```python
from build123d import *

# Parameters (mm, degrees)
SKETCH_1_R          = 1.5
EXTRUDE_1_DEPTH     = 3
CUT_EXTRUDE_1_DEPTH = 182.132548152
FILLET_1_R          = 2


with BuildPart() as part:
    # 草图1 → 凸台-拉伸1 (new body)
    with BuildSketch(Plane(origin=(0, 0, 0), x_dir=(1, 0, 0), z_dir=(0, 1, 0))):
        Polygon((10, -15), (180, -15), (180, 15), (10, 15), (10, 20), (0, 20), (0, -20), (10, -20), align=None)
        with Locations(Location((55, -12, 0), (0, 0, 270))):
            Circle(SKETCH_1_R, mode=Mode.SUBTRACT)
        with Locations(Location((75, -12, 0), (0, 0, 270))):
            Circle(SKETCH_1_R, mode=Mode.SUBTRACT)
        with Locations(Location((3, 15, 0), (0, 0, 270))):
            Circle(SKETCH_1_R, mode=Mode.SUBTRACT)
        with Locations(Location((3, -5, 0), (0, 0, 270))):
            Circle(SKETCH_1_R, mode=Mode.SUBTRACT)
        with Locations(Location((75, 12, 0), (0, 0, 270))):
            Circle(SKETCH_1_R, mode=Mode.SUBTRACT)
        with Locations(Location((55, 12, 0), (0, 0, 270))):
            Circle(SKETCH_1_R, mode=Mode.SUBTRACT)
    extrude(amount=EXTRUDE_1_DEPTH)

    # 草图2 → 切除-拉伸1 (cut, through all)
    with BuildSketch(Plane(origin=(0, 3, 0), x_dir=(1, 0, 0), z_dir=(0, 1, 0))):
        Polygon((20, 10), (10, 0), (20, -10), (25, -10), (15, 0), (25, 10), align=None)
        Polygon((32, -10), (22, 0), (32, 10), (37, 10), (27, 0), (37, -10), align=None)
        Polygon((44, -10), (34, 0), (44, 10), (49, 10), (39, 0), (49, -10), align=None)
        Polygon((50, 0), (58, 8), (63, 8), (55, 0), (63, -8), (58, -8), align=None)
        Polygon((75, -8), (67, 0), (75, 8), (70, 8), (62, 0), (70, -8), align=None)
        Polygon((87, -8), (79, 0), (87, 8), (82, 8), (74, 0), (82, -8), align=None)
        with BuildLine():
            Line((97, 11), (109, 11))
            ThreePointArc((109, 11), (113, 7), (109, 3))
            Line((109, 3), (97, 3))
            ThreePointArc((97, 3), (93, 7), (97, 11))
        make_face()
        with BuildLine():
            Line((97, -11), (109, -11))
            ThreePointArc((109, -11), (113, -7), (109, -3))
            Line((109, -3), (97, -3))
            ThreePointArc((97, -3), (93, -7), (97, -11))
        make_face()
    extrude(amount=-CUT_EXTRUDE_1_DEPTH, mode=Mode.SUBTRACT)

    # 圆角1
    # the kernel refuses this fillet: 2 mm, written as the material it adds along each edge
    with BuildSketch(Plane(origin=(10, 0, -15), x_dir=(1, 0, 0), z_dir=(0, 1, 0)), Plane(origin=(10, 3, 0), x_dir=(0.7071067811865515, 0, -0.7071067811865436), z_dir=(0, -1, 0)), Plane(origin=(34, 3, 0), x_dir=(0.7071067811865507, 0, -0.7071067811865445), z_dir=(0, -1, 0)), Plane(origin=(22, 3, 0), x_dir=(0.7071067811865511, 0, -0.7071067811865441), z_dir=(0, -1, 0)), Plane(origin=(62, 3, 0), x_dir=(0.7071067811865536, 0, -0.7071067811865415), z_dir=(0, -1, 0)), Plane(origin=(74, 3, 0), x_dir=(0.7071067811865546, 0, -0.7071067811865407), z_dir=(0, -1, 0))) as fillet_1_piece_1:
        with BuildLine():
            CenterArc((FILLET_1_R, FILLET_1_R), FILLET_1_R, 180, 90)
            Line((0, FILLET_1_R), (0, 0))
            Line((0, 0), (FILLET_1_R, 0))
        make_face()
    extrude(amount=3)
    with BuildSketch(Plane(origin=(10, 0, 15), x_dir=(1, 0, 0), z_dir=(0, 1, 0)), Plane(origin=(50, 3, 0), x_dir=(0.7071067811865553, 0, 0.7071067811865399), z_dir=(0, -1, 0))) as fillet_1_piece_2:
        with BuildLine():
            CenterArc((FILLET_1_R, -FILLET_1_R), FILLET_1_R, 90, 90)
            Line((0, -FILLET_1_R), (0, 0))
            Line((0, 0), (FILLET_1_R, 0))
        make_face()
    extrude(amount=3)
    with BuildSketch(Plane(origin=(20, 3, -10), x_dir=(-0.7071067811865507, 0, 0.7071067811865442), z_dir=(0, -1, 0)), Plane(origin=(44, 3, 10), x_dir=(1, 0, 0), z_dir=(0, -1, 0)), Plane(origin=(32, 3, 10), x_dir=(1, 0, 0), z_dir=(0, -1, 0))) as fillet_1_piece_3:
        with BuildLine():
            CenterArc((FILLET_1_R * 0.414213562373, -FILLET_1_R), FILLET_1_R, 90, 45)
            Line((-FILLET_1_R * 0.292893218813, -FILLET_1_R * 0.292893218813), (0, 0))
            Line((0, 0), (FILLET_1_R * 0.414213562373, 0))
        make_face()
    extrude(amount=3)
    with BuildSketch(Plane(origin=(20, 3, 10), x_dir=(-0.7071067811865507, 0, -0.7071067811865442), z_dir=(0, -1, 0)), Plane(origin=(44, 3, -10), x_dir=(1, 0, 0), z_dir=(0, -1, 0)), Plane(origin=(32, 3, -10), x_dir=(1, 0, 0), z_dir=(0, -1, 0)), Plane(origin=(70, 3, -8), x_dir=(1, 0, 0), z_dir=(0, -1, 0)), Plane(origin=(70, 3, 8), x_dir=(-0.707106781186555, 0, -0.70710678118654), z_dir=(0, -1, 0)), Plane(origin=(58, 3, 8), x_dir=(-0.7071067811865513, 0, -0.7071067811865438), z_dir=(0, -1, 0)), Plane(origin=(82, 3, -8), x_dir=(1, 0, 0), z_dir=(0, -1, 0)), Plane(origin=(82, 3, 8), x_dir=(-0.7071067811865583, 0, -0.7071067811865369), z_dir=(0, -1, 0)), Plane(origin=(58, 3, -8), x_dir=(1, 0, 0), z_dir=(0, -1, 0))) as fillet_1_piece_4:
        with BuildLine():
            CenterArc((FILLET_1_R * 0.414213562373, FILLET_1_R), FILLET_1_R, 225, 45)
            Line((-FILLET_1_R * 0.292893218813, FILLET_1_R * 0.292893218813), (0, 0))
            Line((0, 0), (FILLET_1_R * 0.414213562373, 0))
        make_face()
    extrude(amount=3)
    with BuildSketch(Plane(origin=(25, 3, 10), x_dir=(-1, 0, 0), z_dir=(0, -1, 0)), Plane(origin=(25, 3, -10), x_dir=(-0.7071067811865513, 0, 0.7071067811865436), z_dir=(0, -1, 0)), Plane(origin=(49, 3, 10), x_dir=(-1, 0, 0), z_dir=(0, -1, 0)), Plane(origin=(49, 3, -10), x_dir=(-0.7071067811865511, 0, 0.7071067811865439), z_dir=(0, -1, 0)), Plane(origin=(37, 3, 10), x_dir=(-1, 0, 0), z_dir=(0, -1, 0)), Plane(origin=(37, 3, -10), x_dir=(-0.707106781186551, 0, 0.707106781186544), z_dir=(0, -1, 0)), Plane(origin=(75, 3, -8), x_dir=(-0.7071067811865541, 0, 0.7071067811865409), z_dir=(0, -1, 0)), Plane(origin=(63, 3, -8), x_dir=(-0.7071067811865546, 0, 0.7071067811865406), z_dir=(0, -1, 0)), Plane(origin=(63, 3, 8), x_dir=(-1, 0, 0), z_dir=(0, -1, 0)), Plane(origin=(87, 3, -8), x_dir=(-0.7071067811865531, 0, 0.7071067811865421), z_dir=(0, -1, 0))) as fillet_1_piece_5:
        with BuildLine():
            CenterArc((FILLET_1_R * 2.41421356237, FILLET_1_R), FILLET_1_R, 135, 135)
            Line((FILLET_1_R * 1.70710678119, FILLET_1_R * 1.70710678119), (0, 0))
            Line((0, 0), (FILLET_1_R * 2.41421356237, 0))
        make_face()
    extrude(amount=3)
    with BuildSketch(Plane(origin=(75, 3, 8), x_dir=(-0.7071067811865545, 0, -0.7071067811865405), z_dir=(0, -1, 0)), Plane(origin=(87, 3, 8), x_dir=(-0.7071067811865538, 0, -0.7071067811865415), z_dir=(0, -1, 0))) as fillet_1_piece_6:
        with BuildLine():
            CenterArc((FILLET_1_R * 2.41421356237, -FILLET_1_R), FILLET_1_R, 90, 135)
            Line((FILLET_1_R * 1.70710678119, -FILLET_1_R * 1.70710678119), (0, 0))
            Line((0, 0), (FILLET_1_R * 2.41421356237, 0))
        make_face()
    extrude(amount=3)
    # the kernel refuses this fillet: 2 mm, written as the material it takes off along each edge
    with BuildSketch(Plane(origin=(10, -5, -20), x_dir=(0, 0, 1), z_dir=(0, 1, 0)), Plane(origin=(180, -5, -15), x_dir=(0, 0, 1), z_dir=(0, 1, 0)), Plane(origin=(180, -5, 15), x_dir=(-1, 0, 0), z_dir=(0, 1, 0)), Plane(origin=(15, 8, 0), x_dir=(0.7071067811865511, 0, 0.707106781186544), z_dir=(0, -1, 0)), Plane(origin=(39, 8, 0), x_dir=(0.7071067811865508, 0, 0.7071067811865444), z_dir=(0, -1, 0)), Plane(origin=(27, 8, 0), x_dir=(0.7071067811865503, 0, 0.7071067811865448), z_dir=(0, -1, 0)), Plane(origin=(67, 8, 0), x_dir=(0.7071067811865541, 0, 0.7071067811865411), z_dir=(0, -1, 0)), Plane(origin=(55, 8, 0), x_dir=(0.7071067811865553, 0, 0.7071067811865397), z_dir=(0, -1, 0)), Plane(origin=(79, 8, 0), x_dir=(0.7071067811865511, 0, 0.7071067811865439), z_dir=(0, -1, 0))) as fillet_1_2_piece_1:
        with BuildLine():
            CenterArc((FILLET_1_R, -FILLET_1_R), FILLET_1_R, 90, 90)
            Line((0, -FILLET_1_R), (0, 0))
            Line((0, 0), (FILLET_1_R, 0))
        make_face()
    extrude(amount=13, mode=Mode.SUBTRACT)
    with BuildSketch(Plane(origin=(10, -5, 20), x_dir=(0, 0, -1), z_dir=(0, 1, 0)), Plane(origin=(0, -5, 20), x_dir=(1, 0, 0), z_dir=(0, 1, 0)), Plane(origin=(0, -5, -20), x_dir=(0, 0, 1), z_dir=(0, 1, 0))) as fillet_1_2_piece_2:
        with BuildLine():
            CenterArc((FILLET_1_R, FILLET_1_R), FILLET_1_R, 180, 90)
            Line((0, FILLET_1_R), (0, 0))
            Line((0, 0), (FILLET_1_R, 0))
        make_face()
    extrude(amount=13, mode=Mode.SUBTRACT)


solid = part.part
```
Source: CAD feature listing. Evaluate the final solid. Frame: model axes, mm. Coordinates: 2 decimals unless noted, no trailing zeros. Loops run counter-clockwise (first coordinate to the right, second up) from the corner with the lowest first, then second, coordinate; pieces in that order, holes last. Notation, with made-up numbers: (14.5, -6) - (57.5, -6) arc R9 ccw to (57.5, -2) - close; hole circle Ø3 at (-35, 49.5). An arc over 180 degrees is marked (long way). Answer as CSV lines item,"result".
1. Ray query, line 1 (X direction, y = 1.65, z = -12); line 2 (Z direction, x = 97.5, y = 0.5); line 3 (X direction, y = 2.85, z = 12.5). Return the intervals inside material, ascending.
Established:
line 1,"x = 0 to 53.5, 56.5 to 73.5, 76.5 to 180"
line 2,"z = -15 to -11, -3 to 3, 11 to 15"
line 3,"x = 0 to 53.59, 56.41 to 73.59, 76.41 to 180"
2. Section A-A (x = 119). Return loops of the section in (y, z).
Established:
outline,"(0, -15) - (3, -15) - (3, 15) - (0, 15) - close"
3. Contact query for flat-ended pins moving along their axis: pin 1 (1 mm diameter, centred on x = 52, y = 2.5, fed in from -Z); pin 2 (1.1 mm diameter, centred on y = 2, z = -17.5, fed in from +X); pin 3 (0.9 mm diameter, centred on x = 61.5, y = 1, fed in from +Z); pin 4 (1.8 mm diameter, centred on x = 3, z = 5, fed in from +Y). Output: stop coordinate, or through.
Established:
pin 1,"stops at z = -15"
pin 2,"stops at x = 10"
pin 3,"stops at z = 15"
pin 4,"passes through"
4. Section B-B (y = 1.3). Count the separate pieces of the cut face and the enclosed holes in it, then the cut area to 3 significant figures.
Established:
separate pieces,"1"
enclosed holes,"14"
area,"4,680 mm2"
